Verification items for this drawing (mm, ordinates from the low corner). Round coordinates to 2 decimals unless told otherwise and drop trailing zeros. Order: outer loops, then holes, each group sorted by start corner. A loop starts at its lowest first (then second) coordinate and runs counter-clockwise, first axis right, second up. Notation, with made-up numbers: (50, 67.5) -> (94, 67.5) arc R29 cw to (94, 94.5) -> close; hole circle Ø7 at (-5.75, 47). An arc over 180 degrees is marked (long way). Return JSON: item names as keys, results as strings. Group by question number.
Item 1: Scan lines: probe 1 along Z at (x, y) = (4, 0.75); probe 2 along Z at (x, y) = (40.5, 0.55); probe 3 along X at (y, z) = (1.1, 45). Record each from-to range of solid material in increasing order. Write a range as from..to.
Item 2: Sectioned sample at A-A on x = 9.5. Record the cut outline in (y, z).
Item 3: Sectioned sample at C-C on z = 46. Record the cut outline in (x, y).
Item 4: Sectioned sample at D-D on x = 25. Record the cut outline in (y, z), plus the area to 3 significant figures.
Item 5: Depth check by flat-ended pin: pin 1 Ø3 at (x, z) = (40.5, 40.5) entering from -Y; pin 2 Ø4 at (x, z) = (40.5, 9.5) entering from +Y; pin 3 Ø6 at (x, z) = (4, 46) entering from +Y. Enter the tip coordinate at first touch or a pass-through.
Item 6: Sectioned sample at B-B on y = 0.95. Give the number of separate pieces and of enclosed holes in the cut face, plus the area to 3 significant figures.
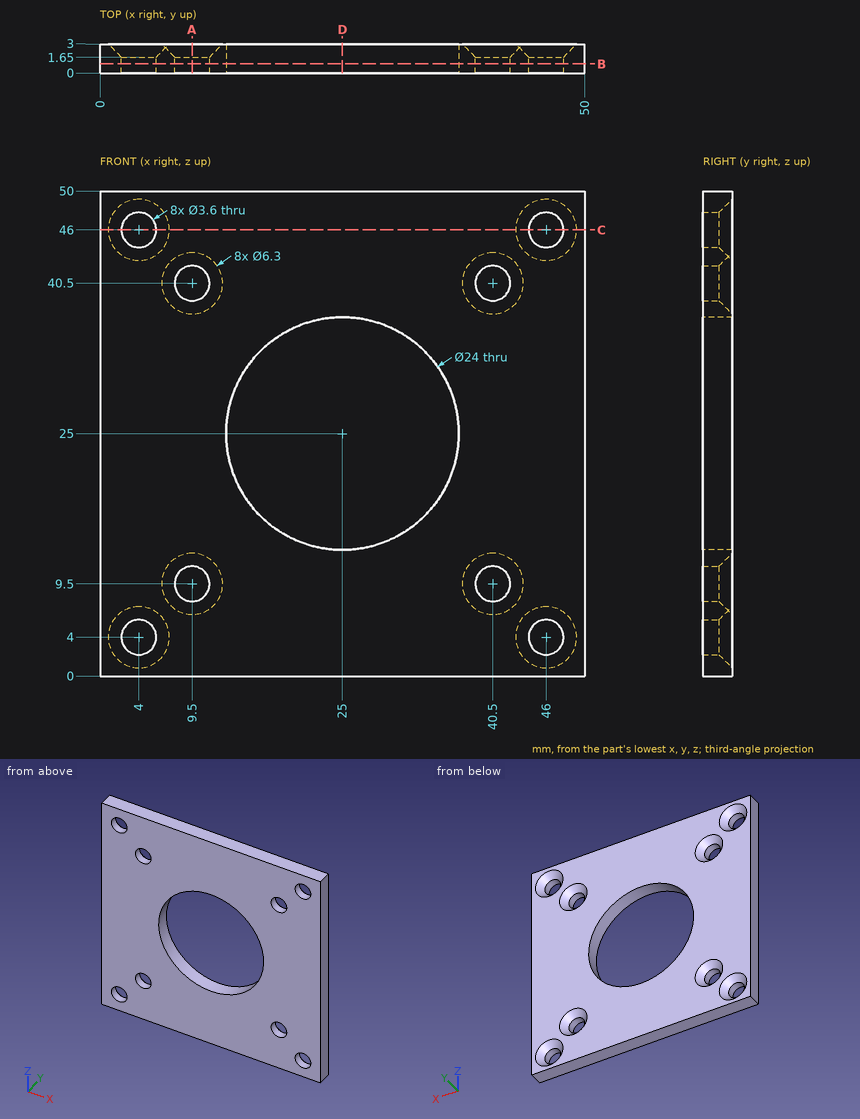
Recorded:
{
 "1": {"probe 1": "0..2.2, 5.8..44.2, 47.8..50", "probe 2": "0..7.7, 11.3..38.7, 42.3..50", "probe 3": "0..2.5, 5.5..44.5, 47.5..50"},
 "2": {"outline": "(0, 0) -> (3, 0) -> (3, 6.35) -> (1.65, 7.7) -> (0, 7.7) -> close; (0, 11.3) -> (1.65, 11.3) -> (3, 12.65) -> (3, 37.35) -> (1.65, 38.7) -> (0, 38.7) -> close; (0, 42.3) -> (1.65, 42.3) -> (3, 43.65) -> (3, 50) -> (0, 50) -> close"},
 "3": {"outline": "(0, 0) -> (2.2, 0) -> (2.2, 1.65) -> (0.85, 3) -> (0, 3) -> close; (5.8, 0) -> (44.2, 0) -> (44.2, 1.65) -> (42.85, 3) -> (7.15, 3) -> (5.8, 1.65) -> close; (47.8, 0) -> (50, 0) -> (50, 3) -> (49.15, 3) -> (47.8, 1.65) -> close"},
 "4": {"outline": "(0, 0) -> (3, 0) -> (3, 13) -> (0, 13) -> close; (0, 37) -> (3, 37) -> (3, 50) -> (0, 50) -> close", "area": "78.0 mm²"},
 "5": {"pin 1": "through", "pin 2": "y = 1.85", "pin 3": "y = 2.85"},
 "6": {"separate pieces": "1", "enclosed holes": "9", "area": "1,970 mm²"}
}
